from build123d import *

# Parameters (mm, degrees)
ESQUISSE1_W              = 55
ESQUISSE1_H              = 43
BOSS_EXTRU_1_DEPTH       = 27
ESQUISSE2_W              = 40.5
ESQUISSE2_H              = 21.676575317
ENL_V_MAT_EXTRU_1_DEPTH  = 38
ESQUISSE3_R              = 0.7
ENL_V_MAT_EXTRU_2_DEPTH  = 43
ESQUISSE4_W              = 55
ESQUISSE4_H              = 20.5
ENL_V_MAT_EXTRU_3_DEPTH  = 11
ENL_V_MAT_EXTRU_6_REACH  = 66.933
ESQUISSE5_W              = 20.5
ESQUISSE5_H              = 10
ESQUISSE6_W              = 7.25
ESQUISSE6_H              = 20.5
ENL_V_MAT_EXTRU_7_DEPTH  = 5
ESQUISSE7_R              = 31
BOSS_EXTRU_2_DEPTH       = 6.5
ESQUISSE8_R              = 41
ESQUISSE8_R_2            = 31
ENL_V_MAT_EXTRU_8_DEPTH  = 6.5
TROU_TARAUD_M2X0_41_D    = 1.6
ESQUISSE10_R             = 10.5
ENL_V_MAT_EXTRU_9_DEPTH  = 4.5
ESQUISSE11_R             = 4.5
ENL_V_MAT_EXTRU_10_DEPTH = 2
ESQUISSE12_R             = 9.25
ESQUISSE12_R_2           = 1.25
BOSS_EXTRU_3_DEPTH       = 5
ESQUISSE13_W             = 50.114904395
ESQUISSE13_H             = 12.012600019
ENL_V_MAT_EXTRU_11_DEPTH = 6.5
BOSS_EXTRU_4_START       = 1.2
BOSS_EXTRU_4_DEPTH       = 1.2
ESQUISSE15_W             = 53.005482756
ESQUISSE15_H             = 10
ENL_V_MAT_EXTRU_12_DEPTH = 7.7
ESQUISSE16_R             = 4.5
ENL_V_MAT_EXTRU_13_DEPTH = 1.2
BOSS_EXTRU_5_START       = -28.2
ESQUISSE17_W             = 40.5
ESQUISSE17_H             = 5
BOSS_EXTRU_5_DEPTH       = 28.2
ESQUISSE18_R             = 1
ENL_V_MAT_EXTRU_14_DEPTH = 10
TROU_TARAUD_M3X0_51_D    = 2.5


with BuildPart() as part:
    # Esquisse1 → Boss.-Extru.1 (new body)
    with BuildSketch(Plane.XY):
        Rectangle(ESQUISSE1_W, ESQUISSE1_H)
    extrude(amount=BOSS_EXTRU_1_DEPTH)

    # Esquisse2 → Enlèv. mat.-Extru.1 (cut)
    with BuildSketch(Plane.XZ.offset(21.5)):
        with Locations((0, 17.338287659)):
            Rectangle(ESQUISSE2_W, ESQUISSE2_H)
    extrude(amount=-ENL_V_MAT_EXTRU_1_DEPTH, mode=Mode.SUBTRACT)

    # Esquisse3 → Enlèv. mat.-Extru.2 (cut)
    with BuildSketch(Plane.XZ.offset(21.5)):
        with Locations(Location((-24.71, 21.675, 0), (0, 0, 270))):
            Circle(ESQUISSE3_R)
        with Locations(Location((-24.71, 11.825, 0), (0, 0, 270))):
            Circle(ESQUISSE3_R)
        with Locations(Location((24.71, 11.825, 0), (0, 0, 270))):
            Circle(ESQUISSE3_R)
        with Locations(Location((24.71, 21.675, 0), (0, 0, 270))):
            Circle(ESQUISSE3_R)
    extrude(amount=-ENL_V_MAT_EXTRU_2_DEPTH, mode=Mode.SUBTRACT)

    # Esquisse4 → Enlèv. mat.-Extru.3 (cut)
    with BuildSketch(Plane.XZ.offset(21.5)):
        with Locations((0, 16.75)):
            Rectangle(ESQUISSE4_W, ESQUISSE4_H)
    extrude(amount=-ENL_V_MAT_EXTRU_3_DEPTH, mode=Mode.SUBTRACT)

    # Enlèv. mat.-Extru.6: up to this face of the body (flat: up to its plane)
    enl_v_mat_extru_6_end = Plane(part.part.faces().sort_by_distance((27.5, 3.85676109, 12.716595404))[0])
    # Esquisse5 → Enlèv. mat.-Extru.6 (cut, up to the picked face)
    with BuildSketch(Plane.ZY.offset(27.5), mode=Mode.PRIVATE) as enl_v_mat_extru_6_sk1:
        with Locations((16.75, 11.5)):
            Rectangle(ESQUISSE5_W, ESQUISSE5_H)
    enl_v_mat_extru_6_tool1 = split(extrude(enl_v_mat_extru_6_sk1.sketch, amount=-ENL_V_MAT_EXTRU_6_REACH, mode=Mode.PRIVATE), bisect_by=enl_v_mat_extru_6_end, keep=Keep.BOTH, mode=Mode.PRIVATE)
    add(enl_v_mat_extru_6_tool1.solids().sort_by(Axis((-27.5, 11.5, 16.75), (1, 0, 0)))[0], mode=Mode.SUBTRACT)

    # Esquisse6 → Enlèv. mat.-Extru.7 (cut)
    with BuildSketch(Plane.XZ.offset(-16.5)):
        with Locations((-23.875, 16.75)):
            Rectangle(ESQUISSE6_W, ESQUISSE6_H)
        with Locations((23.875, 16.75)):
            Rectangle(ESQUISSE6_W, ESQUISSE6_H)
    extrude(amount=-ENL_V_MAT_EXTRU_7_DEPTH, mode=Mode.SUBTRACT)

    # Esquisse7 → Boss.-Extru.2 (add)
    with BuildSketch(Plane(origin=(0, 0, 0), x_dir=(-1, 0, 0), z_dir=(0, 0, -1))):
        Circle(ESQUISSE7_R)
    extrude(amount=-BOSS_EXTRU_2_DEPTH)

    # Esquisse8 → Enlèv. mat.-Extru.8 (cut)
    with BuildSketch(Plane(origin=(0, 0, 0), x_dir=(-1, 0, 0), z_dir=(0, 0, -1))):
        Circle(ESQUISSE8_R)
        Circle(ESQUISSE8_R_2, mode=Mode.SUBTRACT)
    extrude(amount=-ENL_V_MAT_EXTRU_8_DEPTH, mode=Mode.SUBTRACT)

    # Trou taraudé M2x0.41 (through all)
    with Locations(Plane(origin=(-24.71, -10.5, 21.675), x_dir=(0, 0, -1), z_dir=(0, -1, 0))):
        with Locations((0, 0), (9.85, 0), (0, 49.42), (9.85, 49.42)):
            Hole(TROU_TARAUD_M2X0_41_D / 2)

    # Esquisse10 → Enlèv. mat.-Extru.9 (cut)
    with BuildSketch(Plane.XY.offset(6.5)):
        Circle(ESQUISSE10_R)
    extrude(amount=-ENL_V_MAT_EXTRU_9_DEPTH, mode=Mode.SUBTRACT)

    # Esquisse11 → Enlèv. mat.-Extru.10 (cut)
    with BuildSketch(Plane.XY.offset(2)):
        Circle(ESQUISSE11_R)
    extrude(amount=-ENL_V_MAT_EXTRU_10_DEPTH, mode=Mode.SUBTRACT)

    # Esquisse12 → Boss.-Extru.3 (add)
    with BuildSketch(Plane(origin=(0, 21.5, 0), x_dir=(1, 0, 0), z_dir=(0, 1, 0))):
        with Locations(Location((0, -15.876822983, 0), (0, 0, 90))):
            Circle(ESQUISSE12_R)
        with Locations(Location((0, -15.876822983, 0), (0, 0, 270))):
            Circle(ESQUISSE12_R_2, mode=Mode.SUBTRACT)
    extrude(amount=BOSS_EXTRU_3_DEPTH)

    # Esquisse13 → Enlèv. mat.-Extru.11 (cut)
    with BuildSketch(Plane.XY.offset(6.5)):
        with Locations((-0.983340997, 27.50630001)):
            Rectangle(ESQUISSE13_W, ESQUISSE13_H)
    extrude(amount=-ENL_V_MAT_EXTRU_11_DEPTH, mode=Mode.SUBTRACT)

    # Esquisse14 → Boss.-Extru.4 (add)
    with BuildSketch(Plane(origin=(0, 0, 0), x_dir=(-1, 0, 0), z_dir=(0, 0, -1)).offset(BOSS_EXTRU_4_START)):
        with BuildLine():
            Line((-22.332711434, 21.5), (22.332711434, 21.5))
            ThreePointArc((22.332711434, 21.5), (0, -31), (-22.332711434, 21.5))
        make_face()
    extrude(amount=-BOSS_EXTRU_4_DEPTH)

    # Esquisse15 → Enlèv. mat.-Extru.12 (cut)
    with BuildSketch(Plane.XY.offset(6.5)):
        with Locations((0, -26)):
            Rectangle(ESQUISSE15_W, ESQUISSE15_H)
    extrude(amount=-ENL_V_MAT_EXTRU_12_DEPTH, mode=Mode.SUBTRACT)

    # Esquisse16 → Enlèv. mat.-Extru.13 (cut)
    with BuildSketch(Plane.XY):
        Circle(ESQUISSE16_R)
    extrude(amount=-ENL_V_MAT_EXTRU_13_DEPTH, mode=Mode.SUBTRACT)

    # Esquisse17 → Boss.-Extru.5 (add)
    with BuildSketch(Plane.XY.offset(27).offset(BOSS_EXTRU_5_START)):
        with Locations((0, 24)):
            Rectangle(ESQUISSE17_W, ESQUISSE17_H)
    extrude(amount=BOSS_EXTRU_5_DEPTH)

    # Esquisse18 → Enlèv. mat.-Extru.14 (cut)
    with BuildSketch(Plane(origin=(0, 26.5, 0), x_dir=(1, 0, 0), z_dir=(0, 1, 0))):
        with Locations(Location((9.65, -16.5, 0), (0, 0, 270))):
            Circle(ESQUISSE18_R)
    extrude(amount=-ENL_V_MAT_EXTRU_14_DEPTH, mode=Mode.SUBTRACT)

    # Trou taraudé M3x0.51 (through all)
    with Locations(Plane(origin=(9.65, 26.5, 16.5), x_dir=(0, 0, 1), z_dir=(0, 1, 0))):
        with Locations((0, 0)):
            Hole(TROU_TARAUD_M3X0_51_D / 2)


solid = part.part
Input: part model. Units: mm. Frame: model coordinates. A direction names the side the tool comes from. Give positions to 0.01 mm unless a question says otherwise; leave off trailing zeros. Order: outer loops, then holes, each group sorted by start corner. A loop starts at its lowest first (then second) coordinate and runs counter-clockwise, first axis right, second up.
Q1. Ray query, probe 1 along Y at (x, z) = (0, 0.2); probe 2 along Y at (x, z) = (0, 5.1); probe 3 along Z at (x, y) = (24, -6). Return the intervals inside material, ascending.
Checked values:
probe 1: y = -21 to -4.5, 4.5 to 26.5
probe 2: y = -21 to -10.5, 10.5 to 26.5
probe 3: z = -1.2 to 11.46, 12.19 to 21.31, 22.04 to 27
Q2. Section D-D on x = -24.71. Output: boundary loops of the cut face in (y, z) (3 decimals), and give its area (3 significant figures).
Checked values:
outline: (-18.719, -1.2) - (18.719, -1.2) - (18.719, 6.5) - (6.5, 6.5) - (6.5, 11.025) - (-10.5, 11.025) - (-10.5, 6.5) - (-18.719, 6.5) - close; (-10.5, 12.625) - (6.5, 12.625) - (6.5, 20.875) - (-10.5, 20.875) - close; (-10.5, 22.475) - (6.5, 22.475) - (6.5, 27) - (-10.5, 27) - close
area: 582 mm2
Q3. Draft query along X for faces 4 (the flat face through (-20.25, -2, 17)), 5 (the flat face through (27.5, -2, 17)), 6 (the flat face through (-24, -2, 27)). Return one class per face: +X half, -X half, draft (parallel to the pull), parting line (faces both ways), or undercut.
Checked values:
face 4: undercut
face 5: +X half
face 6: draft
Q4. Set-up query: faces 1 (the flat face through (0, 16.5, 17)), 2 (the flat face through (-24, 6.5, 17)), 3 (the flat face through (20.25, -2, 17)). Return all of +Z, -Z, +X, -X, +Y, -Y with unobstructed straight access to the full face (end or side cutting, diameter ignored); none if empty.
Checked values:
face 1: +Z, +X, -X, -Y
face 2: +Z, +X, -X, +Y
face 3: +Z, -Y
Q5. Contact query for flat-ended pins moving along their axis: pin 1 Ø1.5 at (x, y) = (-19.5, -16) entering from +Z; pin 2 Ø8 at (x, z) = (25, 14) entering from +Y; pin 3 Ø6.5 at (x, y) = (0.5, -1.5) entering from +Z. Output: stop coordinate, or through.
Checked values:
pin 1: stops at z = 6.5
pin 2: stops at y = 6.5
pin 3: stops at z = 2
Q6. Section A-A on y = 0. Output: boundary loops of the cut face in (x, z) (3 decimals), and give its area (3 significant figures).
Checked values:
outline: (-31, -1.2) - (-4.5, -1.2) - (-4.5, 2) - (-10.5, 2) - (-10.5, 6.5) - (-20.25, 6.5) - (-20.25, 27) - (-27.5, 27) - (-27.5, 6.5) - (-31, 6.5) - close; (4.5, -1.2) - (31, -1.2) - (31, 6.5) - (27.5, 6.5) - (27.5, 27) - (20.25, 27) - (20.25, 6.5) - (10.5, 6.5) - (10.5, 2) - (4.5, 2) - close; hole circle Ø1.6 at (-24.71, 11.825); hole circle Ø1.6 at (-24.71, 21.675); hole circle Ø1.6 at (24.71, 11.825); hole circle Ø1.6 at (24.71, 21.675)
area: 643 mm2
Q7. Section C-C on x = 0. Output: boundary loops of the cut face in (y, z).
Checked values:
outline: (-21, -1.2) - (-4.5, -1.2) - (-4.5, 2) - (-10.5, 2) - (-10.5, 6.5) - (-21, 6.5) - close; (4.5, -1.2) - (26.5, -1.2) - (26.5, 27) - (16.5, 27) - (16.5, 6.5) - (10.5, 6.5) - (10.5, 2) - (4.5, 2) - close
Q8. Section B-B on z = 16.5. Output: boundary loops of the cut face in (x, y).
Checked values:
outline: (-27.5, -10.5) - (-20.25, -10.5) - (-20.25, 6.5) - (-27.5, 6.5) - close; (-20.25, 16.5) - (8.4, 16.5) - (8.4, 26.5) - (-20.25, 26.5) - close; (10.9, 16.5) - (20.25, 16.5) - (20.25, 26.5) - (10.9, 26.5) - close; (20.25, -10.5) - (27.5, -10.5) - (27.5, 6.5) - (20.25, 6.5) - close
